Autodesk Inventor part; units mm, degrees
ref_plane "1_XY" through (0, 7.112, 0) normal (0, 1, 0) x (1, 0, 0)
ref_plane "1_YZ" through (0, 7.112, 0) normal (1, 0, 0) x (0, 0, -1)
ref_plane "1_ZX" through (0, 7.112, 0) normal (0, 0, -1) x (0, 1, 0)
sketch "Sketch_1" plane through (0, 0, 0) normal (0, 0, 1) x (1, 0, 0)
  line L0 (-3.9497, 0) -> (-3.9497, -6.7945)
  line L1 (-3.9497, -6.7945) -> (-3.6957, -6.7945)
  line L2 (-3.6957, -6.7945) -> (-3.6957, -0.254)
  arc A0 (-3.4417, 0) -> (-3.6957, -0.254) centre (-3.4417, -0.254) ccw
  line L3 (-3.4417, 0) -> (3.4417, 0)
  arc A1 (3.6957, -0.254) -> (3.4417, 0) centre (3.4417, -0.254) ccw
  line L4 (3.6957, -0.254) -> (3.6957, -6.7945)
  line L5 (3.6957, -6.7945) -> (3.9497, -6.7945)
  line L6 (3.9497, -6.7945) -> (3.9497, 0)
  arc A2 (3.9497, 0) -> (3.6957, 0.254) centre (3.6957, 0) ccw
  line L7 (3.6957, 0.254) -> (-3.6957, 0.254)
  arc A3 (-3.6957, 0.254) -> (-3.9497, 0) centre (-3.6957, 0) ccw
extrude "Extrusion1" add sketch "Sketch_1" along normal mid plane 13.0048
sketch "Sketch_2" plane through (0, 0, 0) normal (1, 0, 0) x (0, 1, 0)
  line L0 (0, 7.8029) -> (-9.398, 7.8029)
  line L1 (-9.398, 7.8029) -> (-9.398, -7.8029)
  line L2 (-9.398, -7.8029) -> (0, -7.8029)
  line L3 (0, -7.8029) -> (0, -5.0927)
  line L4 (0, -5.0927) -> (-6.3246, -5.0927)
  line L5 (-6.3246, -5.0927) -> (-6.3246, -2.7305)
  line L6 (-6.3246, -2.7305) -> (-6.6675, -2.7305)
  arc A0 (-6.7945, -2.6035) -> (-6.6675, -2.7305) centre (-6.6675, -2.6035) ccw
  line L7 (-6.7945, -2.6035) -> (-6.7945, -2.0955)
  arc A1 (-6.6675, -1.9685) -> (-6.7945, -2.0955) centre (-6.6675, -2.0955) ccw
  line L8 (-6.6675, -1.9685) -> (-6.3246, -1.9685)
  line L9 (-6.3246, -1.9685) -> (-6.3246, 1.9685)
  line L10 (-6.3246, 1.9685) -> (-6.6675, 1.9685)
  arc A2 (-6.7945, 2.0955) -> (-6.6675, 1.9685) centre (-6.6675, 2.0955) ccw
  line L11 (-6.7945, 2.0955) -> (-6.7945, 2.6035)
  arc A3 (-6.6675, 2.7305) -> (-6.7945, 2.6035) centre (-6.6675, 2.6035) ccw
  line L12 (-6.6675, 2.7305) -> (-6.3246, 2.7305)
  line L13 (-6.3246, 2.7305) -> (-6.3246, 5.0927)
  line L14 (-6.3246, 5.0927) -> (0, 5.0927)
  line L15 (0, 5.0927) -> (0, 7.8029)
extrude "Extrusion2" cut sketch "Sketch_2" along normal mid plane 7.8994
sketch "Sketch_15" plane through (0, 0, 0) normal (0, 0, 1) x (1, 0, 0)
  line L0 (0, 0.127) -> (0, 9.144)
  line L1 (0, 9.144) -> (2.7026, 9.144)
  line L2 (2.7026, 9.144) -> (3.175, 8.6716)
  line L3 (3.175, 8.6716) -> (3.175, 1.143)
  line L4 (3.175, 1.143) -> (4.0005, 1.143)
  line L5 (4.0005, 1.143) -> (4.0005, 0.254)
  line L6 (4.0005, 0.254) -> (2.2225, 0.254)
  line L7 (2.2225, 0.254) -> (2.2225, 0.127)
  line L8 (2.2225, 0.127) -> (0, 0.127)
  line L9 (0, 0.127) -> (0, 9.144)
revolve "Revolution1" add sketch "Sketch_15" angle 360 about axis through (0, 0.127, 0) along (0, -1, 0)
thread "Thread1"
sketch "Sketch_8" plane through (0, 0.254, 0) normal (0, 1, 0) x (1, 0, 0)
  line L0 (-0.3937, 2.4892) -> (0.3937, 2.4892)
  line L1 (0.3937, 2.4892) -> (0.3937, 10.4902)
  line L2 (0.3937, 10.4902) -> (-0.3937, 10.4902)
  line L3 (-0.3937, 10.4902) -> (-0.3937, 2.4892)
extrude "Extrusion3" cut sketch "Sketch_8" along normal blind 9.779
sketch "Sketch_10_ALT_Drilling_1" plane through (0, 0, 0) normal (0, 0, 1) x (1, 0, 0)
  line L0 (0, 0) -> (0, 9.144)
  line L1 (0, 9.144) -> (2.2225, 9.144)
  line L2 (2.2225, 9.144) -> (2.2225, 0)
  line L3 (2.2225, 0) -> (0, 0)
  line L4 (0, 0) -> (0, 9.144)
revolve "Revolution2" cut sketch "Sketch_10_ALT_Drilling_1" angle 360 about axis through (0, 0, 0) along (0, -1, 0)
ref_plane "1_XY" through (0, 7.112, 0) normal (0, 1, 0) x (1, 0, 0)
ref_plane "1_YZ" through (0, 7.112, 0) normal (1, 0, 0) x (0, 0, -1)
ref_plane "1_ZX" through (0, 7.112, 0) normal (0, 0, -1) x (0, 1, 0)
ref_plane "2_XY" through (0, 5.334, 0) normal (0, 1, 0) x (1, 0, 0)
ref_plane "2_YZ" through (0, 5.334, 0) normal (1, 0, 0) x (0, 0, -1)
ref_plane "2_ZX" through (0, 5.334, 0) normal (0, 0, -1) x (0, 1, 0)
ref_plane "3_XY" through (0, 3.556, 0) normal (0, 1, 0) x (1, 0, 0)
ref_plane "3_YZ" through (0, 3.556, 0) normal (1, 0, 0) x (0, 0, -1)
ref_plane "3_ZX" through (0, 3.556, 0) normal (0, 0, -1) x (0, 1, 0)
ref_plane "4_XY" through (0, 2.2225, 0) normal (0, 1, 0) x (1, 0, 0)
ref_plane "4_YZ" through (0, 2.2225, 0) normal (1, 0, 0) x (0, 0, -1)
ref_plane "4_ZX" through (0, 2.2225, 0) normal (0, 0, -1) x (0, 1, 0)
ref_plane "to_base_XY" through (0, 0, 0) normal (0, 1, 0) x (1, 0, 0)
ref_plane "to_base_YZ" through (0, 0, 0) normal (1, 0, 0) x (0, 0, -1)
ref_plane "to_base_ZX" through (0, 0, 0) normal (0, 0, -1) x (0, 1, 0)
properties part number "M201S1M201-bushing"
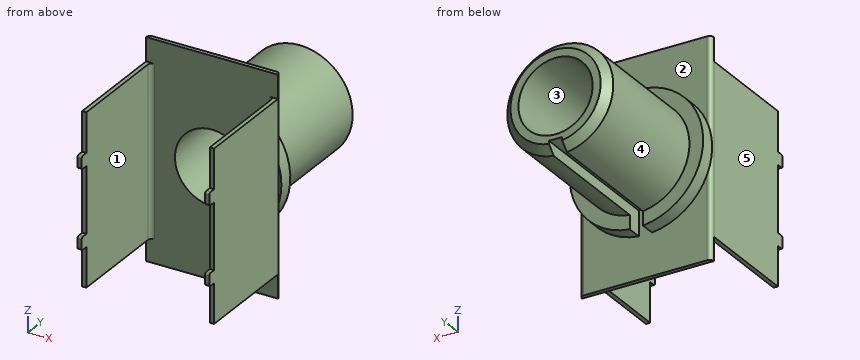
Input: part model. Units: mm. Frame: model coordinates. Face numbers are marked on the shaded views. A direction names the side the tool comes from. Round coordinates to 2 decimals unless told otherwise and drop trailing zeros. Order: outer loops, then holes, each group sorted by start corner. A loop starts at its lowest first (then second) coordinate and runs counter-clockwise, first axis right, second up. Notation, with made-up numbers: (84.5, 69) - (121.5, 69) arc R19 cw to (121.5, 83) - close; hole circle Ø7 at (82.5, 1). An arc over 180 degrees is marked (long way). Answer in a Markdown table with one row per item.
Item 1: Reachability of the marked faces 1 and 2 from +Z, -Z, +X, -X, +Y, -Y: full face, straight path, thin tool, end or side. Return the list, or none.
Model answer:
| item | result |
|---|---|
| face 1 | +Z, -Z, -Y |
| face 2 | +Z, +Y |
Item 2: Mould query, pull axis Z, two halves, no side actions, for the marked faces 3, 4 and 5. Classes: released by +Z, released by -Z, zero draft, split by the parting line, or undercut.
Model answer:
| item | result |
|---|---|
| face 3 | undercut |
| face 4 | split by the parting line |
| face 5 | zero draft |
Item 3: Section query A-A (y = -4.5). Return the cut outline in (x, z), then the cut area to 3 significant figures.
Model answer:
| item | result |
|---|---|
| outline | (-3.95, -5.09) - (-3.7, -5.09) - (-3.7, 5.09) - (-3.95, 5.09) - close; (3.7, -5.09) - (3.95, -5.09) - (3.95, 5.09) - (3.7, 5.09) - close |
| area | 5.17 mm² |
Item 4: Line query: line 1 (X direction, y = -3.5, z = 2.5); line 2 (Z direction, x = 0, y = 4.25) (1 decimal); line 3 (Y direction, x = -2.75, z = 2.5). Output: solid intervals per line, ascending.
Model answer:
| item | result |
|---|---|
| line 1 | x = -3.95 to -3.7, 3.7 to 3.95 |
| line 2 | z = -2.5 to -2.2, 2.2 to 3.2 |
| line 3 | y = 0 to 1.14 |
Item 5: Pin query (flat end, axial travel): pin 1 (0.9 mm diameter, centred on x = 0, y = 3.5, fed in from -Z); pin 2 (1 mm diameter, centred on x = 2.5, z = 4, fed in from -Y); pin 3 (1.5 mm diameter, centred on x = -0.5, z = -4, fed in from +Y). Return the tip coordinate at first contact, or that it passes through.
Model answer:
| item | result |
|---|---|
| pin 1 | stops at z = -3.15 |
| pin 2 | stops at y = 0 |
| pin 3 | stops at y = 1.14 |
